```python
from build123d import *

# Parameters (mm, degrees)
SKETCH_R     = 6.5
PAD_DEPTH    = 22.5
SKETCH001_R  = 4
POCKET_DEPTH = 20
FILLET_R     = 1


with BuildPart() as part:
    # Sketch → Pad (new body)
    with BuildSketch(Plane.XY):
        Circle(SKETCH_R)
    extrude(amount=PAD_DEPTH)

    # Sketch001 (on Face3 of Pad) → Pocket (cut)
    with BuildSketch(Plane.XY.offset(22.5)):
        Circle(SKETCH001_R)
    extrude(amount=-POCKET_DEPTH, mode=Mode.SUBTRACT)

    # Fillet
    fillet_edges = [part.edges().sort_by_distance(p)[0] for p in [
        (6.5, 0, 11.25),
        (-6.5, 0, 0),
        (-6.5, 0, 22.5),
    ]]
    fillet(fillet_edges, radius=FILLET_R)


solid = part.part
```
Input: part model. Units: mm. Frame: model coordinates. Coordinates: 2 decimals unless noted, no trailing zeros. Loops run counter-clockwise (first coordinate to the right, second up) from the corner with the lowest first, then second, coordinate; pieces in that order, holes last.
Q1. Section D-D, the plane z = 2. Return the cut outline in (x, y), and give its area (3 significant figures).
Results are:
outline: circle Ø13 at (0, 0)
area: 133 mm2
Q2. Section A-A, the plane y = 0. Return the cut outline in (x, z).
Results are:
outline: (-6.5, 1) arc R1 ccw to (-5.5, 0) - (5.5, 0) arc R1 ccw to (6.5, 1) - (6.5, 21.5) arc R1 ccw to (5.5, 22.5) - (4, 22.5) - (4, 2.5) - (-4, 2.5) - (-4, 22.5) - (-5.5, 22.5) arc R1 ccw to (-6.5, 21.5) - close
Q3. Contact query for flat-ended pins moving along their axis: pin 1 (6 mm diameter, centred on x = -1.5, y = 3.5, fed in from -Z); pin 2 (5 mm diameter, centred on x = 0, y = 0, fed in from +Z). Output: stop coordinate, or through.
Results are:
pin 1: stops at z = 0
pin 2: stops at z = 2.5
Q4. Section B-B, the plane z = 8. Return the cut outline in (x, y), and give its area (3 significant figures).
Results are:
outline: circle Ø13 at (0, 0); hole circle Ø8 at (0, 0)
area: 82.5 mm2
Q5. Mould query, pull axis Y, two halves, no side actions, for faces 1 (the cylindrical face through (-0.867, -3.905, 12.64)), 2 (the flat face through (0, 0, 2.5)), 3 (the flat face through (-4, -2, 22.5)), 4 (the cylindrical face through (-5.158, -3.955, 11.106)). Classes: +Y half, -Y half, draft (parallel to the pull), parting line (faces both ways), or undercut.
Results are:
face 1: undercut
face 2: undercut
face 3: draft
face 4: parting line
Q6. Line query: line 1 along Y through (x, z) = (0, 16.75); line 2 along Z through (x, y) = (-3.75, 0); line 3 along Y through (x, z) = (-2, 20). Output: solid intervals per line, ascending.
Results are:
line 1: y = -6.5 to -4, 4 to 6.5
line 2: z = 0 to 2.5
line 3: y = -6.18 to -3.46, 3.46 to 6.18
